Read the model definition and answer for the solid it produces. Units are mm, in the model's axes. Face numbers are marked on the shaded views. Round coordinates to 2 decimals unless told otherwise and drop trailing zeros. Write each loop counter-clockwise with the first axis right and the second up, starting at its lowest first coordinate (ties: lowest second). Pieces come first, ordered by that corner, then holes.
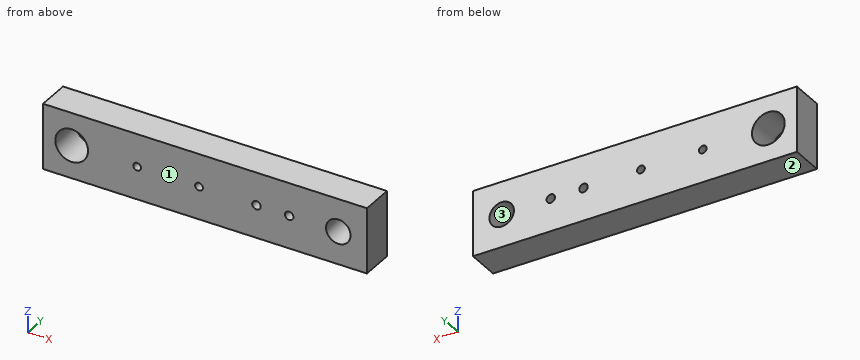
Autodesk Inventor part; units mm, degrees
ref_plane "YZ Plane" through (0, 0, 0) normal (1, 0, 0) x (0, 1, 0)
ref_plane "XZ Plane" through (0, 0, 0) normal (0, 1, 0) x (-1, 0, 0)
ref_plane "XY Plane" through (0, 0, 0) normal (0, 0, 1) x (1, 0, 0)
sketch "Sketch1" plane through (0, 0, 0) normal (1, 0, 0) x (0, 1, 0)
  line L0 (0, 0) -> (12.7, 0)
  line L1 (12.7, 0) -> (12.7, -25.4)
  line L2 (12.7, -25.4) -> (0, -25.4)
  line L3 (0, -25.4) -> (0, 0)
  dimension "d0" = 12.7
  dimension "d1" = 25.4
extrude "Extrusion1" add sketch "Sketch1" along normal blind 125.6538
sketch "Sketch3" plane through (0, 12.7, 0) normal (0, 1, 0) x (1, 0, 0)
  line L0 (0, 0) -> (125.6538, 0)
  line L1 (0, 25.4) -> (125.6538, 25.4)
  circle A0 centre (11.1125, 12.7) radius 6.35
  circle A1 centre (114.5413, 12.7) radius 6.35
  point P0 (36.5125, 12.7)
  point P1 (60.5125, 12.7)
  dimension "d13" = 25.4
  dimension "d14" = 12.7
  dimension "d16" = 24
  dimension "d36" = 25.4
hole "Hole1" at (36.5125, 12.7, -12.7) at (60.5125, 12.7, -12.7) direction (0, -1, 0) diameter 3 end through all
sketch "Sketch5" plane through (0, 12.7, 0) normal (0, 1, 0) x (1, 0, 0)
  line L0 (0, 0) -> (125.6538, 0)
  line L1 (0, 25.4) -> (125.6538, 25.4)
  circle A0 centre (114.5413, 12.7) radius 6.35
  point P0 (95.4913, 12.7)
  dimension "d26" = 12.7
  dimension "d27" = 25.4
  dimension "d28" = 19.05
hole "Hole2" at (95.4913, 12.7, -12.7) direction (0, -1, 0) diameter 3.302 end through all
sketch "Sketch12" plane through (0, 12.7, 0) normal (0, 1, 0) x (1, 0, 0)
  circle A0 centre (95.4913, 12.7) radius 1.651
  circle A1 centre (36.5125, 12.7) radius 1.5
  circle A2 centre (60.5125, 12.7) radius 1.5
  line L0 (0, 0) -> (0, 25.4)
  line L1 (0, 0) -> (125.6538, 0)
  line L2 (125.6538, 25.4) -> (125.6538, 0)
  line L3 (0, 25.4) -> (125.6538, 25.4)
  point P0 (0, 0)
  point P1 (82.7913, 12.7)
  dimension "d77" = 12.7
  dimension "d78" = 12.7
  dimension "d79" = 12.7
hole "Hole5" at (82.7913, 12.7, -12.7) direction (0, -1, 0) diameter 3.302 end through all
sketch "Sketch14" plane through (0, 12.7, 0) normal (0, 1, 0) x (1, 0, 0)
  circle A0 centre (82.7913, 12.7) radius 1.651
  circle A1 centre (95.4913, 12.7) radius 1.651
  circle A2 centre (36.5125, 12.7) radius 1.5
  circle A3 centre (60.5125, 12.7) radius 1.5
  line L0 (0, 0) -> (0, 25.4)
  line L1 (0, 0) -> (125.6538, 0)
  line L2 (125.6538, 25.4) -> (125.6538, 0)
  line L3 (0, 25.4) -> (125.6538, 25.4)
  point P0 (0, 0)
  point P1 (11.1125, 12.7)
hole "Hole7" at (11.1125, 12.7, -12.7) direction (0, -1, 0) diameter 12.7 end through all
sketch "Sketch15" plane through (0, 12.7, 0) normal (0, 1, 0) x (1, 0, 0)
  circle A0 centre (11.1125, 12.7) radius 6.35
  circle A1 centre (82.7913, 12.7) radius 1.651
  circle A2 centre (95.4913, 12.7) radius 1.651
  circle A3 centre (36.5125, 12.7) radius 1.5
  circle A4 centre (60.5125, 12.7) radius 1.5
  line L0 (0, 0) -> (0, 25.4)
  line L1 (0, 0) -> (125.6538, 0)
  line L2 (125.6538, 25.4) -> (125.6538, 0)
  line L3 (0, 25.4) -> (125.6538, 25.4)
  circle A5 centre (114.5413, 12.7) radius 4.7625
  point P0 (0, 0)
hole "Hole8" at (114.5413, 12.7, -12.7) direction (0, -1, 0) diameter 9.525 end through all
properties part number "L17_TSI_005"
Q1. Section B-B (y = 9.5) is taken. State how many separate pieces and enclosed holes the cut face has, then the cut area to 3 significant figures.
Verdict:
separate pieces: 1
enclosed holes: 6
area: 2,960 mm2
Q2. Straight lines are drawn through the part: probe 1 along Z at (x, y) = (115, 7); probe 2 along X at (y, z) = (11.5, -11); probe 3 along X at (y, z) = (10.75, -10.5). For each, find the intervals that lie inside material, in ascending order.
Verdict:
probe 1: z = -25.4 to -17.44, -7.96 to 0
probe 2: x = 0 to 4.99, 17.23 to 110.09, 118.99 to 125.65
probe 3: x = 0 to 5.16, 17.07 to 110.32, 118.77 to 125.65
Q3. Determine the mould class of the marked faces 1, 2 and 3 for opening direction Z: pulls with the +Z half, pulls with the -Z half, needs draft (parallel to the pull), parting line crosses it, or undercut.
Verdict:
face 1: needs draft
face 2: pulls with the -Z half
face 3: undercut
Q4. Section A-A (z = -12.7) is taken. Determine the outline of the cut face in (x, y).
Verdict:
outline: (0, 0) - (4.76, 0) - (4.76, 12.7) - (0, 12.7) - close; (17.46, 0) - (35.01, 0) - (35.01, 12.7) - (17.46, 12.7) - close; (38.01, 0) - (59.01, 0) - (59.01, 12.7) - (38.01, 12.7) - close; (62.01, 0) - (81.14, 0) - (81.14, 12.7) - (62.01, 12.7) - close; (84.44, 0) - (93.84, 0) - (93.84, 12.7) - (84.44, 12.7) - close; (97.14, 0) - (109.78, 0) - (109.78, 12.7) - (97.14, 12.7) - close; (119.3, 0) - (125.65, 0) - (125.65, 12.7) - (119.3, 12.7) - close
